Autodesk Inventor part; units mm, degrees
ref_plane "YZ Plane" through (0, 0, 0) normal (1, 0, 0) x (0, 1, 0)
ref_plane "XZ Plane" through (0, 0, 0) normal (0, 1, 0) x (-1, 0, 0)
ref_plane "XY Plane" through (0, 0, 0) normal (0, 0, 1) x (1, 0, 0)
sketch "Sketch1" plane through (0, 0, 0) normal (0, 0, 1) x (1, 0, 0)
  line L0 (0, 0) -> (-30, 0)
  line L1 (-30, 0) -> (-30, 8)
  line L2 (-30, 8) -> (0, 8)
  line L3 (0, 8) -> (0, 0)
  line L4 (0, 8) -> (-30, 8)
  line L5 (-30, 8) -> (-30, -92)
  line L6 (-30, -92) -> (0, -92)
  line L7 (0, -92) -> (0, 8)
  dimension "d0" = 30
  dimension "d1" = 8
  dimension "d2" = 100
extrude "Extrusion1" add sketch "Sketch1" along normal blind 3
sketch "Sketch2" plane through (0, 0, 0) normal (0, 0, -1) x (-1, 0, 0)
  line L0 (30, 8) -> (30, -92)
  line L1 (0, -92) -> (0, 8)
  line L2 (30, 8) -> (0, 8)
  line L3 (0, 8) -> (0, 5)
  line L4 (0, 5) -> (30, 5)
  line L5 (30, 5) -> (30, 8)
  point P0 (0, 0)
  point P1 (0, 8)
  dimension "d5" = 3
extrude "Extrusion2" add sketch "Sketch2" along normal blind 42
sketch "Sketch3" plane through (-30, 8, 3) normal (0, 1, 0) x (1, 0, 0)
  line L0 (0, 45) -> (0, 0)
  line L1 (0, 45) -> (0, 30)
  line L2 (0, 30) -> (10, 30)
  circle A0 centre (10, 30) radius 2.5
  line L3 (30, 0) -> (30, 45)
  line L4 (30, 45) -> (30, 30)
  circle A1 centre (20, 30) radius 2.5
  point P0 (30, 3)
  dimension "d8" = 15
  dimension "d9" = 10
  dimension "d10" = 5
  dimension "d11" = 15
  dimension "d12" = 5
  dimension "d13" = 10
extrude "Extrusion3" cut sketch "Sketch3" against normal blind 42
sketch "Sketch4" plane through (0, 0, 0) normal (0, 0, -1) x (-1, 0, 0)
  circle A0 centre (15, -62) radius 6.35
  line L0 (30, -92) -> (0, -92)
  line L1 (0, -92) -> (0, 5)
  point P0 (0, 0)
  dimension "d16" = 12.7
  dimension "d17" = 30
  dimension "d18" = 15
extrude "Extrusion4" cut sketch "Sketch4" against normal blind 42
sketch "Sketch5" plane through (-30, 8, 3) normal (0, 1, 0) x (1, 0, 0)
  point P0 (30, 3)
sketch "Sketch6" plane through (-30, 8, 3) normal (0, 1, 0) x (1, 0, 0)
  point P0 (30, 3)
properties part number "Angle"
Part model, mm, in its own coordinate system. A direction names the side the tool comes from. Coordinates: 2 decimals unless noted, no trailing zeros. Loops run counter-clockwise (first coordinate to the right, second up) from the corner with the lowest first, then second, coordinate; pieces in that order, holes last. Notation, with made-up numbers: (4, -7) -> (10, -7) arc R22 ccw to (10, 10) -> close; hole circle Ø7 at (-30.5, 66). An arc over 180 degrees is marked (long way). Use a Markdown table: item, result. Add a question column.
Item 1: Band-saw the part on C-C on z = -27. Write the cut outline in (x, y).
Item 2: Band-saw the part on A-A on y = -62. Write the cut outline in (x, z).
Item 3: Pull direction Z, two halves, no side cores. Call faces 3 (the flat face through (-15, -41, 3)), 4 (the cylindrical face through (-21.84, 6.52, -28.69)), 5 (the flat face through (-15, 7, -42)), 6 (the cylindrical face through (-13.62, -68.2, 1.48)): +Z half, -Z half, draft (parallel to the pull), parting line (faces both ways), or undercut.
Item 4: Which spindle directions (+Z, -Z, +X, -X, +Y, -Y) get a long thin tool onto all of the face, cutting with end or side? Do faces 1 (the flat face through (-15, -92, 1)), 2 (the flat face through (-15, 5, -21)). Say none if no direction does.
Item 5: Band-saw the part on D-D on x = -10. Write the cut outline in (y, z).
Item 6: Band-saw the part on B-B on x = -15. Write the cut outline in (y, z).
Item 7: Flat gauge pins, fed straight in: P1, Ø4, axis at x = -11.5, z = -13, coming from the -Y side; P2, Ø9, axis at x = -12.5, y = -55, coming from the -Z side. Where does each tip first touch, or does it go through?
Item 8: Probe probe 1 along X at (y, z) = (6, -27); probe 2 along Z at (x, y) = (-20, 5.7); probe 3 along Y at (x, z) = (-15, 2.1). List the from-to ranges inside material, lowest first.
Geometry says:
| question | item | result |
|---|---|---|
| 1 | outline | (-30, 5) -> (-22.5, 5) -> (-22.5, 8) -> (-30, 8) -> close; (-17.5, 5) -> (-12.5, 5) -> (-12.5, 8) -> (-17.5, 8) -> close; (-7.5, 5) -> (0, 5) -> (0, 8) -> (-7.5, 8) -> close |
| 2 | outline | (-30, 0) -> (-21.35, 0) -> (-21.35, 3) -> (-30, 3) -> close; (-8.65, 0) -> (0, 0) -> (0, 3) -> (-8.65, 3) -> close |
| 3 | face 3 | +Z half |
| 3 | face 4 | undercut |
| 3 | face 5 | -Z half |
| 3 | face 6 | draft |
| 4 | face 1 | +Z, -Z, +X, -X, -Y |
| 4 | face 2 | -Z, +X, -X, -Y |
| 5 | outline | (-92, 0) -> (-65.91, 0) -> (-65.91, 3) -> (-92, 3) -> close; (-58.09, 0) -> (5, 0) -> (5, -24.5) -> (8, -24.5) -> (8, 3) -> (-58.09, 3) -> close; (5, -42) -> (8, -42) -> (8, -29.5) -> (5, -29.5) -> close |
| 6 | outline | (-92, 0) -> (-68.35, 0) -> (-68.35, 3) -> (-92, 3) -> close; (-55.65, 0) -> (5, 0) -> (5, -42) -> (8, -42) -> (8, 3) -> (-55.65, 3) -> close |
| 7 | P1 | y = 5 |
| 7 | P2 | z = 0 |
| 8 | probe 1 | -30 to -22.5, -17.5 to -12.5, -7.5 to 0 |
| 8 | probe 2 | -42 to -29.5, -24.5 to 3 |
| 8 | probe 3 | -92 to -68.35, -55.65 to 8 |
